Check sheet for the modelled part. Datum: model origin and axes. Units: mm. Face numbers are marked on the shaded views. A direction names the side the tool comes from. Coordinates: 2 decimals unless noted, no trailing zeros. Write each loop counter-clockwise with the first axis right and the second up, starting at its lowest first coordinate (ties: lowest second). Pieces come first, ordered by that corner, then holes. Notation, with made-up numbers: (14.25, 47.5) - (53.25, 47.5) arc R21 ccw to (53.25, 53.5) - close; hole circle Ø4 at (3, -15.5). An arc over 180 degrees is marked (long way). Use one line per item in the form item = value. Start each with the question number.
1. Scan lines: line 1 along X through (y, z) = (7.75, -20); line 2 along Z through (x, y) = (45, 11); line 3 along Z through (x, y) = (-18, 15.25). Record each from-to range of solid material in increasing order.
2. Cross-section at B-B on y = 6.5. Give the number of separate pieces and of enclosed holes in the cut face, then the cut area to 3 significant figures.
3. Tool access check on the marked faces 4 and 5. Record the directions out of +Z, -Z, +X, -X, +Y, -Y that give a thin tool (end or side, any length) a straight path to the whole face; none if there is none.
4. Draft check along Z on the marked faces 1, 2 and 3. Enter one of: +Z half, -Z half, draft (parallel to the pull), parting line (faces both ways), or undercut.
5. Go/stop test with flat-tipped pins: pin 1 Ø7 at (x, z) = (-18, -20) entering from +Y; pin 2 Ø14.5 at (x, z) = (45, 20) entering from +Y; pin 3 Ø6.5 at (x, z) = (18, 20) entering from +Y. Record where each tip stops, or that it passes through.
6. Cross-section at A-A on x = 45. Record the boundary of the cut face in (y, z), then the cut area to 3 significant figures.
```python
from build123d import *

# Parameters (mm, degrees)
DODANIE_WYCI_GNI_CIE1_DEPTH                       = 20
OTWORY_USTALAJ_CE_8_0MM1_D                        = 8
OTWORY_USTALAJ_CE_8_0MM1_DEPTH                    = 15
OTWORY_USTALAJ_CE_8_0MM1_TIP                      = 2.403442476
POG_BIENIE_WALCOWE_POD_M8_RUB_Z_BEM_S_D           = 9
POG_BIENIE_WALCOWE_POD_M8_RUB_Z_BEM_S_CBORE_D     = 18.011
POG_BIENIE_WALCOWE_POD_M8_RUB_Z_BEM_S_CBORE_DEPTH = 5.3


with BuildPart() as part:
    # Szkic1 → Dodanie-wyciągnięcie1 (new body)
    with BuildSketch(Plane(origin=(0, 0, 0), x_dir=(1, 0, 0), z_dir=(0, 1, 0))):
        with BuildLine():
            Line((-52.5, -40), (52.5, -40))
            ThreePointArc((52.5, -40), (59.571067812, -37.071067812), (62.5, -30))
            Line((62.5, -30), (62.5, 30))
            ThreePointArc((62.5, 30), (59.571067812, 37.071067812), (52.5, 40))
            Line((52.5, 40), (-52.5, 40))
            ThreePointArc((-52.5, 40), (-59.571067812, 37.071067812), (-62.5, 30))
            Line((-62.5, 30), (-62.5, -30))
            ThreePointArc((-62.5, -30), (-59.571067812, -37.071067812), (-52.5, -40))
        make_face()
    extrude(amount=DODANIE_WYCI_GNI_CIE1_DEPTH)

    # Otwory ustalające Ø8.0mm1
    with Locations(Plane(origin=(0, 20, 0), x_dir=(1, 0, 0), z_dir=(0, 1, 0))):
        with Locations((-18, -20), (18, -20), (18, 20), (-18, 20)):
            Hole(OTWORY_USTALAJ_CE_8_0MM1_D / 2, depth=OTWORY_USTALAJ_CE_8_0MM1_DEPTH)
            with Locations((0, 0, -(OTWORY_USTALAJ_CE_8_0MM1_DEPTH + OTWORY_USTALAJ_CE_8_0MM1_TIP / 2))):  # 118° drill point
                Cone(0, OTWORY_USTALAJ_CE_8_0MM1_D / 2, OTWORY_USTALAJ_CE_8_0MM1_TIP, mode=Mode.SUBTRACT)

    # Pogłębienie walcowe pod M8 śrubę z łbem szeciokątnym1 (through all)
    with Locations(Plane(origin=(0, 20, 0), x_dir=(1, 0, 0), z_dir=(0, 1, 0))):
        with Locations((-45, 20), (-45, -20), (45, -20), (45, 20)):
            CounterBoreHole(POG_BIENIE_WALCOWE_POD_M8_RUB_Z_BEM_S_D / 2, POG_BIENIE_WALCOWE_POD_M8_RUB_Z_BEM_S_CBORE_D / 2, POG_BIENIE_WALCOWE_POD_M8_RUB_Z_BEM_S_CBORE_DEPTH)


solid = part.part
```
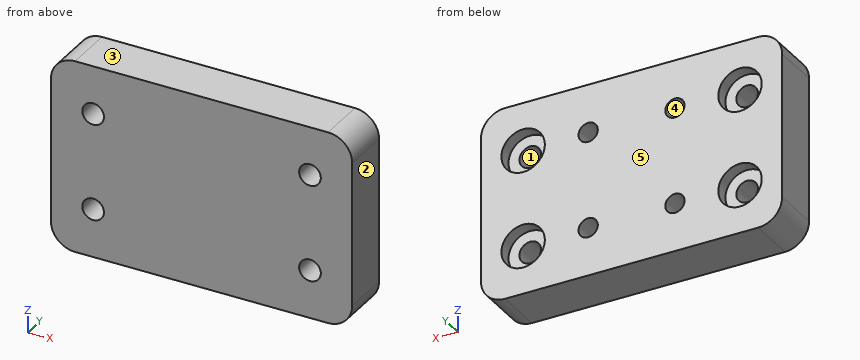
Final values:
q1.line_1 = -62.5 to -49.5, -40.5 to -22, -14 to 14, 22 to 40.5, 49.5 to 62.5
q1.line_2 = -40 to -24.5, -15.5 to 15.5, 24.5 to 40
q1.line_3 = -40 to -24, -16 to 16, 24 to 40
q2.separate_pieces = 1
q2.enclosed_holes = 8
q2.area = 9,460 mm²
q3.face_4 = +Y
q3.face_5 = +Z, -Z, +X, -X, +Y
q4.face_1 = undercut
q4.face_2 = draft
q4.face_3 = +Z half
q5.pin_1 = 4.7
q5.pin_2 = 14.7
q5.pin_3 = 4.55
q6.outline = (0, -40) - (20, -40) - (20, -29.01) - (14.7, -29.01) - (14.7, -24.5) - (0, -24.5) - close; (0, -15.5) - (14.7, -15.5) - (14.7, -10.99) - (20, -10.99) - (20, 10.99) - (14.7, 10.99) - (14.7, 15.5) - (0, 15.5) - close; (0, 24.5) - (14.7, 24.5) - (14.7, 29.01) - (20, 29.01) - (20, 40) - (0, 40) - close
q6.area = 1,140 mm²
